```python
from build123d import *

# Parameters (mm, degrees)
CROQUIS1_W              = 25
CROQUIS1_H              = 10
CROQUIS1_R              = 2
SALIENTE_EXTRUIR1_DEPTH = 4
CROQUIS2_W              = 6.835109388
CROQUIS2_H              = 13
SALIENTE_EXTRUIR2_DEPTH = 24
CROQUIS3_R              = 2
CORTAR_EXTRUIR1_DEPTH   = 24
SALIENTE_EXTRUIR3_DEPTH = 4
CORTAR_EXTRUIR2_DEPTH   = 24


with BuildPart() as part:
    # Croquis1 → Saliente-Extruir1 (new body)
    with BuildSketch(Plane(origin=(0, 0, 0), x_dir=(0, 0, -1), z_dir=(1, 0, 0))):
        with Locations((7.35898106, 5.127314815)):
            Rectangle(CROQUIS1_W, CROQUIS1_H)
        with Locations((1.05898106, 5.127314815)):
            Circle(CROQUIS1_R, mode=Mode.SUBTRACT)
        with Locations((13.55898106, 5.127314815)):
            Circle(CROQUIS1_R, mode=Mode.SUBTRACT)
    extrude(amount=SALIENTE_EXTRUIR1_DEPTH)

    # Croquis2 → Saliente-Extruir2 (add)
    with BuildSketch(Plane(origin=(4, 0, 0), x_dir=(0, 0, -1), z_dir=(1, 0, 0))):
        with Locations((7.35898106, 3.627314815)):
            Rectangle(CROQUIS2_W, CROQUIS2_H)
    extrude(amount=SALIENTE_EXTRUIR2_DEPTH)

    # Croquis3 → Cortar-Extruir1 (cut)
    with BuildSketch(Plane(origin=(0, 10.127314815, 0), x_dir=(1, 0, 0), z_dir=(0, 1, 0))):
        with Locations(Location((22, 7.35898106, 0), (0, 0, 270))):
            Circle(CROQUIS3_R)
    extrude(amount=-CORTAR_EXTRUIR1_DEPTH, mode=Mode.SUBTRACT)

    # Croquis4 → Saliente-Extruir3 (add, through all)
    with BuildSketch(Plane(origin=(4, 0, 0), x_dir=(0, 0, -1), z_dir=(1, 0, 0))):
        Polygon((-5.14101894, 0.127314815), (3.941426366, -2.872685185), (10.776535754, -2.872685185), (19.85898106, 0.127314815), align=None)
    extrude(amount=-SALIENTE_EXTRUIR3_DEPTH)

    # Croquis5 → Cortar-Extruir2 (cut)
    with BuildSketch(Plane(origin=(0, 10.127314815, 0), x_dir=(1, 0, 0), z_dir=(0, 1, 0))):
        with BuildLine():
            Line((28, 3.941426366), (24.720702874, 3.941426366))
            ThreePointArc((24.720702874, 3.941426366), (26.368283898, 7.35898106), (24.720702874, 10.776535754))
            Line((24.720702874, 10.776535754), (28, 10.776535754))
            Line((28, 10.776535754), (28, 3.941426366))
        make_face()
    extrude(amount=-CORTAR_EXTRUIR2_DEPTH, mode=Mode.SUBTRACT)


solid = part.part
```
Here's how the part is built. I have some questions about the finished solid (model axes, mm). A direction names the side the tool comes from. Coordinates: 2 decimals unless noted, no trailing zeros. Loops run counter-clockwise (first coordinate to the right, second up) from the corner with the lowest first, then second, coordinate; pieces in that order, holes last. Notation, with made-up numbers: (-28.5, -25) - (26.5, -25) arc R21 ccw to (26.5, -4) - close; hole circle Ø6 at (-26.5, 9.25). An arc over 180 degrees is marked (long way). Return JSON: item names as keys, results as strings. Group by question number.
Item 1: If we section it at C-C on z = -15.25: Write out the boundary of the cut face in (x, y).
Item 2: Will these pins go through, and if not, where does the flat tip stop? P1, Ø3.5, axis at x = 22, z = -7.36, coming from the -Y side; P2, Ø6, axis at x = 15, y = 3.5, coming from the +Z side; P3, Ø7.5, axis at y = 3.5, z = -15.5, coming from the +X side; P4, Ø1, axis at x = 12, y = 8.5, coming from the -Z side.
Item 3: On a 3-axis mill with a long thin cutter (end or side, diameter ignored), from which of +Z, -Z, +X, -X, +Y, -Y can I reach the whole of each face in a straight line? I mean faces 5 (the face through (4, 3.7, -15.3)), 6 (the face through (2.028, -1.352, 0.663)), 7 (the face through (4, 4, 1)). Say none if no direction works.
Item 4: If we section it at A-A on x = 22: Write out the boundary of the cut face in (y, z).
Item 5: I need wall thicknesses on line 1 (X direction, y = 0.25, z = -7.5); line 2 (Z direction, x = 6.75, y = 2.5); line 3 (X direction, y = 8.5, z = -3.75). Which ranges of each line are inside material? Lowest first, please. Write a range as from..to.
Item 6: We'd pull the mould along Y, two halves only. Please class faces 1 (the face through (1.97, 7.11, -0.8)), 2 (the face through (20.783, 3.718, -8.946)), 3 (the face through (1.972, 6.814, -14.634)), 4 (the face through (2.028, -1.394, -15.254)): +Y half, -Y half, draft (parallel to the pull), parting line (faces both ways), or undercut.
Item 7: If we section it at D-D on x = 2.75: Write out the boundary of the cut face in (y, z).
Item 8: If we section it at B-B on y = 8.5: Write out the boundary of the cut face in (x, z), and give its area (3 significant figures).
Calculated:
{
 "1": {"outline": "(0, -1.4) - (4, -1.4) - (4, 4.06) - (0, 4.06) - close; (0, 6.2) - (4, 6.2) - (4, 10.13) - (0, 10.13) - close"},
 "2": {"P1": "passes through", "P2": "stops at z = -3.94", "P3": "stops at x = 4", "P4": "stops at z = -10.78"},
 "3": {"face 5": "-Z, +X, +Y, -Y", "face 6": "+Z, +X, -X, -Y", "face 7": "+Z, +X, +Y, -Y"},
 "4": {"outline": "(-2.87, -10.78) - (10.13, -10.78) - (10.13, -9.36) - (-2.87, -9.36) - close; (-2.87, -5.36) - (10.13, -5.36) - (10.13, -3.94) - (-2.87, -3.94) - close"},
 "5": {"line 1": "x = 0..20, 24..26.37", "line 2": "z = -10.78..-3.94", "line 3": "x = 0..4"},
 "6": {"face 1": "undercut", "face 2": "draft", "face 3": "undercut", "face 4": "-Y half"},
 "7": {"outline": "(-2.87, -10.78) - (0.13, -19.86) - (10.13, -19.86) - (10.13, 5.14) - (0.13, 5.14) - (-2.87, -3.94) - close; hole circle Ø4 at (5.13, -13.56); hole circle Ø4 at (5.13, -1.06)"},
 "8": {"outline": "(0, -19.86) - (4, -19.86) - (4, -10.78) - (24.72, -10.78) arc R4.37 ccw to (24.72, -3.94) - (4, -3.94) - (4, 5.14) - (0, 5.14) - close; hole circle Ø4 at (22, -7.36)", "area": "237 mm^2"}
}
